Model file for the job. Use its own axes, mm. A direction names the side the tool comes from. Give positions to 0.01 mm unless a question says otherwise; leave off trailing zeros. Order: outer loops, then holes, each group sorted by start corner. A loop starts at its lowest first (then second) coordinate and runs counter-clockwise, first axis right, second up. Notation, with made-up numbers: (-14.5, 16) - (12.5, 16) arc R35 cw to (12.5, 48) - close; hole circle Ø7 at (44, 17.5). An arc over 180 degrees is marked (long way). Return JSON: item names as keys, results as strings. Group by question number.
from build123d import *

# Parameters (mm, degrees)
PAD_DEPTH = 1.8


with BuildPart() as pad:
    # Sketch001 → Pad (new body, symmetric)
    with BuildSketch(Plane.YZ):
        with BuildLine():
            Line((4, 0), (4, 10))
            Line((4, 10), (6.5, 10))
            Line((6.5, 10), (9.53921, 15.635917))
            ThreePointArc((16.703013, 10.339192), (16.175328, 17.118372), (9.53921, 15.635917))
            Line((6.5, 0), (16.703013, 10.339192))
            Line((4, 0), (6.5, 0))
        make_face()
        with BuildLine():
            Line((-16.703013, 10.339192), (-6.5, 0))
            Line((-6.5, 0), (-4, 0))
            Line((-4, 0), (-4, 10))
            Line((-4, 10), (-6.5, 10))
            Line((-6.5, 10), (-9.53921, 15.635917))
            ThreePointArc((-9.53921, 15.635917), (-16.175328, 17.118372), (-16.703013, 10.339192))
        make_face()
    extrude(amount=PAD_DEPTH, both=True)


with BuildPart() as obj1:
    # Sketch → Revolution (revolve)
    with BuildSketch(Plane.YZ):
        Polygon((4, 0), (3.325, 0.389711), (3.325, 9.610289), (4, 10), (5.5, 10), (6.5, 0), align=None)
    revolve(axis=Axis((0, 0, 0), (0, 0, 1)))

    # Fusion: union Pad
    add(pad.part)


solid = obj1.part
(1) Slice it at D-D (z = 13.5). Give the cut face in (x, y), and give its area (3 significant figures).
(2) Slice it at B-B (y = 0). Give the cut face in (x, z) (3 decimals).
(3) Slice it at A-A (x = 0). Give the cut face in (y, z) (3 decimals).
(4) Slice it at C-C (z = 3). Give the cut face in (x, y) (3 decimals), and give its area (3 significant figures).
(5) 3-axis set-ups, long thin cutter, end or side, ignore diameter. For faces 4 (the face through (3, -3, 10)), 5 (the face through (6, 0, 5)): which of +Z, -Z, +X, -X, +Y, -Y reach the whole face in a straight line?
(6) Drill centre lines: L1, parallel to Y at x = 0, z = 5.75 (3 decimals); L2, parallel to Y at x = 0.5, z = 11; L3, parallel to X at y = 13, z = 15.5. Where is each one in solid material? Low to high.
(7) Pull direction X, two halves, no side cores. Call faces 1 (the face through (2.95, 1.53, 5.06)), 2 (the face through (0.03, -16.09, 17.18)), 3 (the face through (1.8, 12, 11)): released by +X, released by -X, zero draft, split by the parting line, or undercut.
(8) Drop flat-ended pins along their axis: pin 1 Ø6 at (x, y) = (0.5, 2.5) entering from +Z; pin 2 Ø10 at (y, z) = (8.5, 9.5) entering from -X; pin 3 Ø7.5 at (x, y) = (0, 0) entering from -Z; pin 4 Ø3 at (x, z) = (5, 14) entering from -Y. Give the stop position or say it passes through.
Result set:
{
 "1": {"outline": "(-1.8, -18) - (1.8, -18) - (1.8, -8.39) - (-1.8, -8.39) - close; (-1.8, 8.39) - (1.8, 8.39) - (1.8, 18) - (-1.8, 18) - close", "area": "69.2 mm²"},
 "2": {"outline": "(-6.5, 0) - (-4, 0) - (-3.325, 0.39) - (-3.325, 9.61) - (-4, 10) - (-5.5, 10) - close; (3.325, 0.39) - (4, 0) - (6.5, 0) - (5.5, 10) - (4, 10) - (3.325, 9.61) - close"},
 "3": {"outline": "(-16.703, 10.339) - (-6.5, 0) - (-4, 0) - (-3.325, 0.39) - (-3.325, 9.61) - (-4, 10) - (-6.5, 10) - (-9.539, 15.636) arc R4.5 ccw (long way) to start; (3.325, 0.39) - (4, 0) - (6.5, 0) - (16.703, 10.339) arc R4.5 ccw (long way) to (9.539, 15.636) - (6.5, 10) - (4, 10) - (3.325, 9.61) - close"},
 "4": {"outline": "(-1.8, -9.46) - (1.8, -9.46) - (1.8, -5.933) arc R6.2 ccw to (1.8, 5.933) - (1.8, 9.46) - (-1.8, 9.46) - (-1.8, 5.933) arc R6.2 ccw to (-1.8, -5.933) - close; hole circle Ø6.65 at (0, 0)", "area": "110 mm²"},
 "5": {"face 4": "+Z, +X, -X", "face 5": "+Z, +X"},
 "6": {"L1": "y = -12.174 to -3.325, 3.325 to 12.174", "L2": "y = -17.24 to -7.04, 7.04 to 17.24", "L3": "x = -1.8 to 1.8"},
 "7": {"face 1": "undercut", "face 2": "zero draft", "face 3": "released by +X"},
 "8": {"pin 1": "stops at z = 10", "pin 2": "stops at x = -4.36", "pin 3": "stops at z = 0.14", "pin 4": "passes through"}
}
